```python
from build123d import *

# Parameters (mm, degrees)
SKETCH_1_R          = 13
SKETCH_1_R_2        = 11
EXTRUDE_1_DEPTH     = 600
SKETCH_2_W          = 2
SKETCH_2_H          = 30
CUT_EXTRUDE_1_DEPTH = 14


with BuildPart() as part:
    # 草图1 → 凸台-拉伸1 (new body)
    with BuildSketch(Plane(origin=(0, 0, 0), x_dir=(1, 0, 0), z_dir=(0, 1, 0))):
        Circle(SKETCH_1_R)
        Circle(SKETCH_1_R_2, mode=Mode.SUBTRACT)
    extrude(amount=EXTRUDE_1_DEPTH)

    # 草图2 → 切除-拉伸1 (cut, through all)
    with BuildSketch(Plane(origin=(0, 0, 0), x_dir=(0, 0, -1), z_dir=(1, 0, 0))):
        with Locations((0, 585)):
            Rectangle(SKETCH_2_W, SKETCH_2_H)
        with Locations((0, 15)):
            Rectangle(SKETCH_2_W, SKETCH_2_H)
    extrude(amount=-CUT_EXTRUDE_1_DEPTH, mode=Mode.SUBTRACT)


solid = part.part
```
For this review, take the finished solid that the model builds, in its own axes (mm). Give positions to 0.01 mm unless a question says otherwise; leave off trailing zeros. Order: outer loops, then holes, each group sorted by start corner. A loop starts at its lowest first (then second) coordinate and runs counter-clockwise, first axis right, second up.
1) Take a section at B-B (z = 6.5). Give the boundary of the cut face in (x, y), then the cut area to 3 significant figures.
2) Wall thickness on line 1 (Z direction, x = 0, y = 383.5); line 2 (Z direction, x = -8.5, y = 488): over which ranges is each line inside the solid? List them lowest first.
3) Take a section at C-C (y = 492). Give the boundary of the cut face in (x, z).
4) Insertion check: pin 1 (3 mm diameter, centred on y = 462.5, z = 6.5, fed in from +X); pin 2 (3 mm diameter, centred on y = 339, z = -3, fed in from -X); pin 3 (2 mm diameter, centred on x = -12, y = 11.5, fed in from +Z); pin 4 (6 mm diameter, centred on x = 1.5, z = -6, fed in from +Y). Each pin has a flat end and moves straight along its axis. Give the tip position at first contact, or say it passes through.
5) The part is to be moulded in two halves that separate along X. For faces 1 (the face through (12.4, 295.8, -3.9)), 2 (the face through (3, 600, -11)), 3 (the face through (10.161, 295.8, 4.213)), say which applies: released by +X, released by -X, zero draft, split by the parting line, or undercut.
6) Take a section at A-A (x = 0). Give the boundary of the cut face in (y, z).
Derived:
1. outline: (-11.26, 0) - (-8.87, 0) - (-8.87, 600) - (-11.26, 600) - close; (8.87, 0) - (11.26, 0) - (11.26, 600) - (8.87, 600) - close
1. area: 2,860 mm2
2. line 1: z = -13 to -11, 11 to 13
2. line 2: z = -9.84 to -6.98, 6.98 to 9.84
3. outline: circle Ø26 at (0, 0); hole circle Ø22 at (0, 0)
4. pin 1: stops at x = 12
4. pin 2: stops at x = -12.91
4. pin 3: stops at z = 6.93
4. pin 4: passes through
5. face 1: split by the parting line
5. face 2: zero draft
5. face 3: undercut
6. outline: (0, -13) - (600, -13) - (600, -11) - (0, -11) - close; (0, 11) - (600, 11) - (600, 13) - (0, 13) - close
